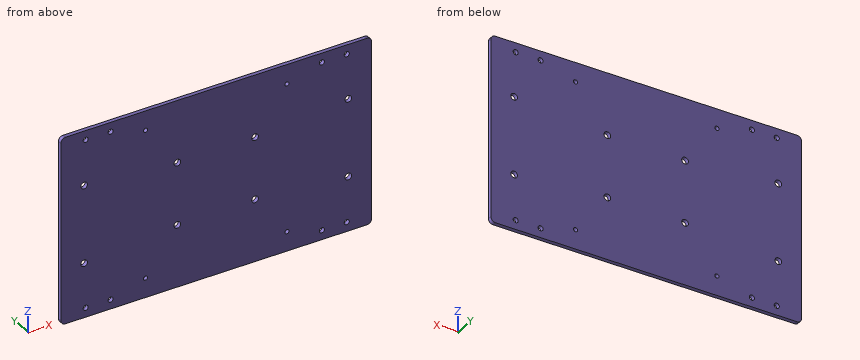
from build123d import *

# Parameters (mm, degrees)
SKETCH_1_W          = 200
SKETCH_1_H          = 120
SKETCH_1_R          = 1.65
SKETCH_1_R_2        = 2.15
EXTRUDE_2_DEPTH     = 2.5
CUT_EXTRUDE_1_REACH = 118.646
SKETCH_2_R          = 1.35
FILLET_1_R          = 3


with BuildPart() as part:
    # 草圖1 → 填料-伸長2 (new body)
    with BuildSketch(Plane(origin=(0, 0, 0), x_dir=(1, 0, 0), z_dir=(0, 1, 0))):
        Rectangle(SKETCH_1_W, SKETCH_1_H)
        with Locations(Location((-84, 54, 0), (0, 0, 270))):
            Circle(SKETCH_1_R, mode=Mode.SUBTRACT)
        with Locations(Location((-68, 54, 0), (0, 0, 270))):
            Circle(SKETCH_1_R, mode=Mode.SUBTRACT)
        with Locations(Location((68, 54, 0), (0, 0, 270))):
            Circle(SKETCH_1_R, mode=Mode.SUBTRACT)
        with Locations(Location((84, 54, 0), (0, 0, 270))):
            Circle(SKETCH_1_R, mode=Mode.SUBTRACT)
        with Locations(Location((84, -54, 0), (0, 0, 90))):
            Circle(SKETCH_1_R, mode=Mode.SUBTRACT)
        with Locations(Location((68, -54, 0), (0, 0, 90))):
            Circle(SKETCH_1_R, mode=Mode.SUBTRACT)
        with Locations(Location((-68, -54, 0), (0, 0, 90))):
            Circle(SKETCH_1_R, mode=Mode.SUBTRACT)
        with Locations(Location((-84, -54, 0), (0, 0, 90))):
            Circle(SKETCH_1_R, mode=Mode.SUBTRACT)
        with Locations(Location((25, 20, 0), (0, 0, 270))):
            Circle(SKETCH_1_R_2, mode=Mode.SUBTRACT)
        with Locations(Location((-25, 20, 0), (0, 0, 270))):
            Circle(SKETCH_1_R_2, mode=Mode.SUBTRACT)
        with Locations(Location((-25, -20, 0), (0, 0, 270))):
            Circle(SKETCH_1_R_2, mode=Mode.SUBTRACT)
        with Locations(Location((25, -20, 0), (0, 0, 270))):
            Circle(SKETCH_1_R_2, mode=Mode.SUBTRACT)
        with Locations(Location((85, 25, 0), (0, 0, 270))):
            Circle(SKETCH_1_R_2, mode=Mode.SUBTRACT)
        with Locations(Location((85, -25, 0), (0, 0, 270))):
            Circle(SKETCH_1_R_2, mode=Mode.SUBTRACT)
        with Locations(Location((-85, -25, 0), (0, 0, 90))):
            Circle(SKETCH_1_R_2, mode=Mode.SUBTRACT)
        with Locations(Location((-85, 25, 0), (0, 0, 90))):
            Circle(SKETCH_1_R_2, mode=Mode.SUBTRACT)
    extrude(amount=EXTRUDE_2_DEPTH)

    # 草圖2 → 除料-伸長1 (cut, up to next)
    with BuildSketch(Plane(origin=(0, 2.5, 0), x_dir=(1, 0, 0), z_dir=(0, 1, 0)), mode=Mode.PRIVATE) as cut_extrude_1_sk1:
        with Locations(Location((-45.5, 47.5, 0), (0, 0, 270))):
            Circle(SKETCH_2_R)
    cut_extrude_1_tool1 = extrude(cut_extrude_1_sk1.sketch, amount=-CUT_EXTRUDE_1_REACH, mode=Mode.PRIVATE) & part.part
    # 草圖2 → 除料-伸長1 (cut, up to next)
    with BuildSketch(Plane(origin=(0, 2.5, 0), x_dir=(1, 0, 0), z_dir=(0, 1, 0)), mode=Mode.PRIVATE) as cut_extrude_1_sk2:
        with Locations(Location((45.5, 47.5, 0), (0, 0, 270))):
            Circle(SKETCH_2_R)
    cut_extrude_1_tool2 = extrude(cut_extrude_1_sk2.sketch, amount=-CUT_EXTRUDE_1_REACH, mode=Mode.PRIVATE) & part.part
    # 草圖2 → 除料-伸長1 (cut, up to next)
    with BuildSketch(Plane(origin=(0, 2.5, 0), x_dir=(1, 0, 0), z_dir=(0, 1, 0)), mode=Mode.PRIVATE) as cut_extrude_1_sk3:
        with Locations(Location((-45.5, -47.5, 0), (0, 0, 270))):
            Circle(SKETCH_2_R)
    cut_extrude_1_tool3 = extrude(cut_extrude_1_sk3.sketch, amount=-CUT_EXTRUDE_1_REACH, mode=Mode.PRIVATE) & part.part
    # 草圖2 → 除料-伸長1 (cut, up to next)
    with BuildSketch(Plane(origin=(0, 2.5, 0), x_dir=(1, 0, 0), z_dir=(0, 1, 0)), mode=Mode.PRIVATE) as cut_extrude_1_sk4:
        with Locations(Location((45.5, -47.5, 0), (0, 0, 270))):
            Circle(SKETCH_2_R)
    cut_extrude_1_tool4 = extrude(cut_extrude_1_sk4.sketch, amount=-CUT_EXTRUDE_1_REACH, mode=Mode.PRIVATE) & part.part
    add(cut_extrude_1_tool1.solids().sort_by_distance((-45.5, 2.5, -47.5))[0], mode=Mode.SUBTRACT)
    add(cut_extrude_1_tool2.solids().sort_by_distance((45.5, 2.5, -47.5))[0], mode=Mode.SUBTRACT)
    add(cut_extrude_1_tool3.solids().sort_by_distance((-45.5, 2.5, 47.5))[0], mode=Mode.SUBTRACT)
    add(cut_extrude_1_tool4.solids().sort_by_distance((45.5, 2.5, 47.5))[0], mode=Mode.SUBTRACT)

    # 圓角1
    fillet_1_edges = [part.edges().sort_by_distance(p)[0] for p in [
        (-100, 1.25, -60),
        (100, 1.25, -60),
        (100, 1.25, 60),
        (-100, 1.25, 60),
    ]]
    fillet(fillet_1_edges, radius=FILLET_1_R)


solid = part.part
The model under review builds one solid part; all positions refer to its coordinate system, in mm. Round coordinates to 2 decimals unless told otherwise and drop trailing zeros. Write each loop counter-clockwise with the first axis right and the second up, starting at its lowest first coordinate (ties: lowest second). Pieces come first, ordered by that corner, then holes. Notation, with made-up numbers: (22.25, 5) - (33.25, 5) arc R15 cw to (33.25, 12) - close; hole circle Ø10 at (40, 20). An arc over 180 degrees is marked (long way). One line per item, written item: value. Start each with the question number.
1. Consider section A-A on z = -20. Write out the cut boundary in (x, y), and give its area (4 significant figures).
2. To check wall thickness, follow L1, parallel to X at y = 1.85, z = 54; L2, parallel to Z at x = -24, y = 2.3; L3, parallel to Z at x = -85, y = 2. State the ranges of each line that lie inside material, in increasing order. Write a range as from..to.
3. Consider section B-B on x = -25. Write out the cut boundary in (y, z), and give its area (4 significant figures).
Checks:
1. outline: (-100, 0) - (-27.15, 0) - (-27.15, 2.5) - (-100, 2.5) - close; (-22.85, 0) - (22.85, 0) - (22.85, 2.5) - (-22.85, 2.5) - close; (27.15, 0) - (100, 0) - (100, 2.5) - (27.15, 2.5) - close
1. area: 478.5 mm^2
2. L1: x = -100..-85.65, -82.35..-69.65, -66.35..66.35, 69.65..82.35, 85.65..100
2. L2: z = -60..-21.9, -18.1..18.1, 21.9..60
2. L3: z = -60..-55.31, -52.69..-27.15, -22.85..22.85, 27.15..52.69, 55.31..60
3. outline: (0, -60) - (2.5, -60) - (2.5, -22.15) - (0, -22.15) - close; (0, -17.85) - (2.5, -17.85) - (2.5, 17.85) - (0, 17.85) - close; (0, 22.15) - (2.5, 22.15) - (2.5, 60) - (0, 60) - close
3. area: 278.5 mm^2
